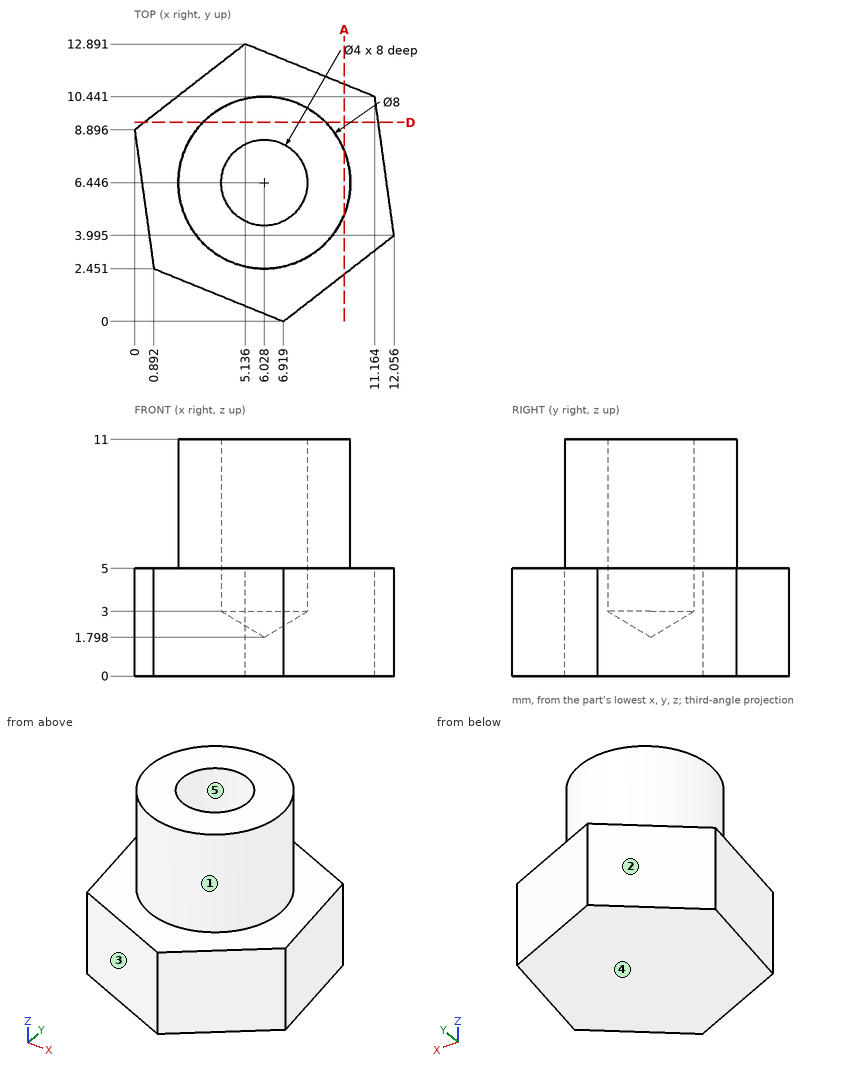
The drawing under review shows one solid part. Ordinate dimensions are in mm from its lowest x, y, z. A direction names the side the tool comes from. Round coordinates to 2 decimals unless told otherwise and drop trailing zeros. Write each loop counter-clockwise with the first axis right and the second up, starting at its lowest first coordinate (ties: lowest second). Pieces come first, ordered by that corner, then holes.
(1) Mouldability with a two-part tool opening along Y and no side actions: class the marked faces 3, 4 and 5 as +Y half, -Y half, draft (parallel to the pull), parting line (faces both ways), or undercut.
(2) Machinability: for the marked faces 1 and 2, which of the approach directions +Z, -Z, +X, -X, +Y, -Y give a long, thin tool a straight path to every point of the face, cutting with its end or side? Answer none if there is none.
(3) Insertion check: pin 1 (5 mm diameter, centred on y = 4.5, z = 3, fed in from -X); pin 2 (3 mm diameter, centred on y = 3.5, z = 1, fed in from +X); pin 3 (1.5 mm diameter, centred on x = 3.5, z = 4, fed in from -Y) (1 decimal); pin 4 (2 mm diameter, centred on y = 9.5, z = 7.5, fed in from +X). Each pin has a flat end and moves straight along its axis. Give the tip position at first contact, or say it passes through.
(4) We need section D-D on y = 9.25. Give the boundary of the cut face in (x, z) (1 decimal).
(5) We need section A-A on x = 9.75. Give the boundary of the cut face in (y, z) (1 decimal).
(6) Wall thickness on L1, parallel to X at y = 6.5, z = 6.5; L2, parallel to Y at x = 5.5, z = 9.5 (1 decimal); L3, parallel to Z at x = 6.75, y = 11.25: over which ranges is each line inside the solid? List them lowest first.
Findings below:
1. face 3: -Y half
1. face 4: draft
1. face 5: undercut
2. face 1: +Z
2. face 2: +Z, -Z, -X, +Y
3. pin 1: stops at x = 0.26
3. pin 2: stops at x = 12.06
3. pin 3: stops at y = 1.1
3. pin 4: stops at x = 9.46
4. outline: (0.5, 0) - (11.3, 0) - (11.3, 5) - (8.9, 5) - (8.9, 11) - (3.2, 11) - (3.2, 5) - (0.5, 5) - close
5. outline: (2.2, 0) - (11, 0) - (11, 5) - (7.9, 5) - (7.9, 11) - (5, 11) - (5, 5) - (2.2, 5) - close
6. L1: x = 2.03 to 4.03, 8.03 to 10.03
6. L2: y = 2.5 to 4.5, 8.4 to 10.4
6. L3: z = 0 to 5
